```python
from build123d import *

# Parameters (mm, degrees)
SKETCH_1_W          = 7.5
SKETCH_1_H          = 4
SKETCH_2_R          = 1.75
CUT_EXTRUDE_1_DEPTH = 5


with BuildPart() as part:
    # 草圖1 → 旋轉1 (revolve)
    with BuildSketch(Plane(origin=(0, 0, 0), x_dir=(1, 0, 0), z_dir=(0, 1, 0))):
        Polygon((0, 30), (0, 0), (5, 0), (5, 4), (5, 30), align=None)
        with Locations((8.75, 2)):
            Rectangle(SKETCH_1_W, SKETCH_1_H)
    revolve(axis=Axis((0, 0, 0), (0, 0, -1)))

    # 草圖2 → 除料-伸長1 (cut, through all)
    with BuildSketch(Plane(origin=(0, 0, -4), x_dir=(-1, 0, 0), z_dir=(0, 0, -1))):
        with Locations((0, 10)):
            Circle(SKETCH_2_R)
        with Locations((8.660254038, 5)):
            Circle(SKETCH_2_R)
        with Locations((8.660254038, -5)):
            Circle(SKETCH_2_R)
        with Locations((0, -10)):
            Circle(SKETCH_2_R)
        with Locations((-8.660254038, -5)):
            Circle(SKETCH_2_R)
        with Locations((-8.660254038, 5)):
            Circle(SKETCH_2_R)
    extrude(amount=-CUT_EXTRUDE_1_DEPTH, mode=Mode.SUBTRACT)


solid = part.part
```
The model under review builds one solid part; all positions refer to its coordinate system, in mm. A direction names the side the tool comes from. Round coordinates to 2 decimals unless told otherwise and drop trailing zeros. Order: outer loops, then holes, each group sorted by start corner. A loop starts at its lowest first (then second) coordinate and runs counter-clockwise, first axis right, second up. Notation, with made-up numbers: (2, 25.5) - (38, 25.5) arc R21 ccw to (38, 43.5) - close; hole circle Ø4 at (34, -39.75). An arc over 180 degrees is marked (long way). Answer in a Markdown table with one row per item.
(1) Take a section at B-B on y = 10. Write out the cut boundary in (x, z), plus the area to 3 significant figures.
Result set:
| item | result |
|---|---|
| outline | (-7.5, -4) - (-1.75, -4) - (-1.75, 0) - (-7.5, 0) - close; (1.75, -4) - (7.5, -4) - (7.5, 0) - (1.75, 0) - close |
| area | 46.0 mm2 |
(2) Take a section at A-A on x = 0. Write out the cut boundary in (y, z).
Result set:
| item | result |
|---|---|
| outline | (-12.5, -4) - (-11.75, -4) - (-11.75, 0) - (-12.5, 0) - close; (-8.25, -4) - (-5, -4) - (-5, -30) - (5, -30) - (5, -4) - (8.25, -4) - (8.25, 0) - (-8.25, 0) - close; (11.75, -4) - (12.5, -4) - (12.5, 0) - (11.75, 0) - close |
(3) Take a section at C-C on z = -3.25. Write out the cut boundary in (x, y).
Result set:
| item | result |
|---|---|
| outline | circle Ø25 at (0, 0); hole circle Ø3.5 at (-8.66, -5); hole circle Ø3.5 at (-8.66, 5); hole circle Ø3.5 at (0, -10); hole circle Ø3.5 at (0, 10); hole circle Ø3.5 at (8.66, -5); hole circle Ø3.5 at (8.66, 5) |
(4) Mouldability with a two-part tool opening along X and no side actions: class faces 1 (the face through (0, 0, 0)), 2 (the face through (0.228, -8.265, -2.028)), 3 (the face through (11.923, -3.755, -2.028)) as released by +X, released by -X, zero draft, split by the parting line, or undercut.
Result set:
| item | result |
|---|---|
| face 1 | zero draft |
| face 2 | undercut |
| face 3 | split by the parting line |
(5) Clearance check with flat-ended pins moving along their axes: P1, Ø10, axis at x = 1.5, z = -11, coming from the +Y side; P2, Ø5, axis at x = 9, z = -26.5, coming from the -Y side; P3, Ø4.5, axis at x = 0, y = -10, coming from the -Z side; P4, Ø6, axis at y = 7, z = -26, coming from the -X side. State where each tip first meets the part, or that it passes through.
Result set:
| item | result |
|---|---|
| P1 | stops at y = 5 |
| P2 | passes through |
| P3 | stops at z = -4 |
| P4 | stops at x = -3 |
(6) Machinability: for faces 4 (the face through (0.2, 5.4, -4)), 5 (the face through (0, 0, -30)), which of the approach directions +Z, -Z, +X, -X, +Y, -Y give a long, thin tool a straight path to every point of the face, cutting with its end or side? Answer none if there is none.
Result set:
| item | result |
|---|---|
| face 4 | -Z |
| face 5 | -Z, +X, -X, +Y, -Y |
(7) For line 1 (Y direction, x = 0, z = -2.45); line 2 (Z direction, x = -4.75, y = 5.5); line 3 (Y direction, x = -8.25, z = -3.25), list the stretches that pass through material, from the lowest coordinate up. Write a range as from..to.
Result set:
| item | result |
|---|---|
| line 1 | y = -12.5..-11.75, -8.25..8.25, 11.75..12.5 |
| line 2 | z = -4..0 |
| line 3 | y = -9.39..-6.7, -3.3..3.3, 6.7..9.39 |
(8) Take a section at D-D on x = 7.75. Write out the cut boundary in (y, z), plus the area to 3 significant figures.
Result set:
| item | result |
|---|---|
| outline | (-9.81, -4) - (-6.49, -4) - (-6.49, 0) - (-9.81, 0) - close; (-3.51, -4) - (3.51, -4) - (3.51, 0) - (-3.51, 0) - close; (6.49, -4) - (9.81, -4) - (9.81, 0) - (6.49, 0) - close |
| area | 54.5 mm2 |
